Here's how the part is built. I have some questions about the finished solid (model axes, mm). Face numbers are marked on the shaded views. A direction names the side the tool comes from. Give positions to 0.01 mm unless a question says otherwise; leave off trailing zeros. Loops run counter-clockwise (first coordinate to the right, second up) from the corner with the lowest first, then second, coordinate; pieces in that order, holes last.
Q1. If we section it at A-A (x = 31.5): Please give me the cut outline in (y, z), plus the area to 3 significant figures.
Q2. If we section it at D-D (y = 4): Please give me the cut outline in (x, z), plus the area to 4 significant figures.
Q3. For the marked faces 1, 2, 3, 4 and 5, which set-ups out of +Z, -Z, +X, -X, +Y, -Y let a thin tool reach every point of the face, with its end or its side?
Q4. Will these pins go through, and if not, where does the flat tip stop? P1, Ø1, axis at x = -2.5, y = -1, coming from the -Z side; P2, Ø5, axis at x = -9, y = 23.5, coming from the -Z side; P3, Ø2, axis at y = 18, z = -5, coming from the -X side.
Q5. I need wall thicknesses on line 1 (X direction, y = 22.5, z = -0.5); line 2 (Z direction, x = -3, y = -17); line 3 (Y direction, x = 28, z = -13.75). Which ranges of each line are inside material? Lowest first, please.
Q6. If we section it at C-C (z = -12.5): Please give me the cut outline in (x, y).
Q7. If we section it at B-B (y = 20.5): Please give me the cut outline in (x, z).
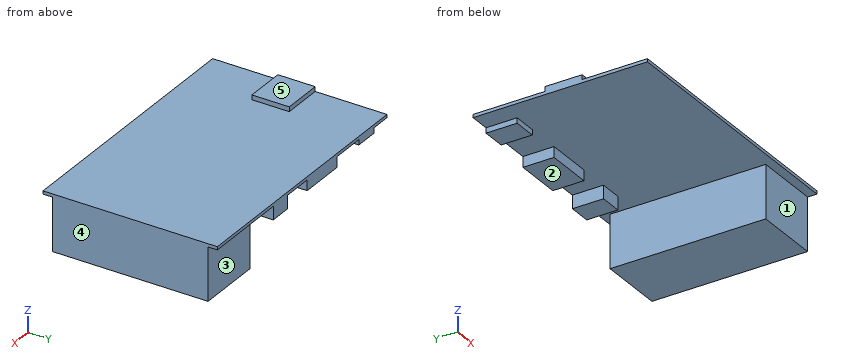
Autodesk Inventor part; units mm, degrees
ref_plane "YZ Plane" through (0, 0, 0) normal (1, 0, 0) x (0, 1, 0)
ref_plane "XZ Plane" through (0, 0, 0) normal (0, 1, 0) x (-1, 0, 0)
ref_plane "XY Plane" through (0, 0, 0) normal (0, 0, 1) x (1, 0, 0)
sketch "Sketch1" plane through (0, 0, 0) normal (0, 0, 1) x (1, 0, 0)
  line L0 (42.5, -28) -> (-42.5, -28)
  line L1 (-42.5, -28) -> (-42.5, 28)
  line L2 (-42.5, 28) -> (42.5, 28)
  line L3 (42.5, 28) -> (42.5, -28)
  line L4 (42.5, -28) -> (-42.5, 28) construction
  line L5 (-42.5, -28) -> (42.5, 28) construction
  point P0 (0, 0)
  dimension "d0" = 85
  dimension "d1" = 56
extrude "Extrusion1" add sketch "Sketch1" along normal blind 1
sketch "Sketch2" plane through (42.5, -28, 0) normal (1, 0, 0) x (0, 0, -1)
  line L0 (0, 56) -> (0, 0)
  line L1 (0, 53) -> (17, 53)
  line L2 (17, 53) -> (17, 3)
  line L3 (17, 3) -> (0, 3)
  line L4 (0, 3) -> (0, 53)
  line L5 (0, 56) -> (-1, 56)
  line L6 (0, 0) -> (-1, 0)
  point P0 (0, 28)
  dimension "d4" = 3
  dimension "d5" = 3
  dimension "d6" = 17
extrude "Extrusion2" add sketch "Sketch2" against normal blind 21
sketch "Sketch3" plane through (-42.5, 28, 0) normal (0, 1, 0) x (1, 0, 0)
  line L0 (49.8, 0) -> (57, 0)
  line L1 (57, 0) -> (57, 4.2398)
  line L2 (57, 4.2398) -> (49.8, 4.2398)
  line L3 (49.8, 4.2398) -> (49.8, 0)
  line L4 (25, 0) -> (40, 0)
  line L5 (40, 0) -> (40, 3.3654)
  line L6 (40, 3.3654) -> (25, 3.3654)
  line L7 (25, 3.3654) -> (25, 0)
  line L8 (6.5, 1.6827) -> (14.1, 1.6827)
  line L9 (14.1, 1.6827) -> (14.1, 0)
  line L10 (14.1, 0) -> (6.5, 0)
  line L11 (6.5, 0) -> (6.5, 1.6827)
  line L12 (85, 0) -> (85, -1)
  line L13 (0, 0) -> (0, -1)
  point P0 (42.5, 0)
  dimension "d9" = 28
  dimension "d10" = 7.2
  dimension "d11" = 6.5
  dimension "d12" = 7.6
  dimension "d13" = 15
  dimension "d14" = 25
extrude "Extrusion3" add sketch "Sketch3" against normal blind 10
sketch "Sketch4" plane through (0, 0, 1) normal (0, 0, 1) x (1, 0, 0)
  line L0 (-42.5, -7.0526) -> (-29.5, -7.0526)
  line L1 (-29.5, -7.0526) -> (-29.5, 4.9474)
  line L2 (-29.5, 4.9474) -> (-42.5, 4.9474)
  line L3 (-42.5, 4.9474) -> (-42.5, -7.0526)
  line L4 (-42.5, 28) -> (-42.5, -28)
  point P0 (0, 0)
  dimension "d17" = 12
  dimension "d18" = 13
extrude "Extrusion4" add sketch "Sketch4" along normal blind 1.5
properties part number "Raspi"
Check sheet entries:
1. outline: (-28, 0) - (-25, 0) - (-25, -17) - (25, -17) - (25, 0) - (28, 0) - (28, 1) - (-28, 1) - close
1. area: 906 mm2
2. outline: (-42.5, 0) - (21.5, 0) - (21.5, -17) - (42.5, -17) - (42.5, 1) - (-29.5, 1) - (-29.5, 2.5) - (-42.5, 2.5) - close
2. area: 461.5 mm2
3. face 1: -Z, +X, -X, -Y
3. face 2: -Z, -X, +Y, -Y
3. face 3: -Z, +X, +Y
3. face 4: +Z, -Z, +X, +Y, -Y
3. face 5: +Z, +X, -X, +Y, -Y
4. P1: stops at z = 0
4. P2: stops at z = -3.37
4. P3: stops at x = 7.3
5. line 1: x = -36 to -28.4, -17.5 to -2.5, 7.3 to 14.5, 21.5 to 42.5
5. line 2: z = 0 to 1
5. line 3: y = -25 to 25
6. outline: (21.5, -25) - (42.5, -25) - (42.5, 25) - (21.5, 25) - close
7. outline: (-42.5, 0) - (-36, 0) - (-36, -1.68) - (-28.4, -1.68) - (-28.4, 0) - (-17.5, 0) - (-17.5, -3.37) - (-2.5, -3.37) - (-2.5, 0) - (7.3, 0) - (7.3, -4.24) - (14.5, -4.24) - (14.5, 0) - (21.5, 0) - (21.5, -17) - (42.5, -17) - (42.5, 1) - (-42.5, 1) - close
